```python
from build123d import *

# Parameters (mm, degrees)
F1_DEPTH = 6.35
F2_R     = 3.175
F3_DEPTH = 6.35
F5_DEPTH = 6.35
F4_R     = 22.225
F4_R_2   = 19.05
F6_DEPTH = 25.4


with BuildPart() as f1:
    # F0 (on Top) → F1 (new body)
    with BuildSketch(Plane.XY):
        Polygon((-42.868439, 12.7), (-42.868439, 0), (-42.868439, -12.7), (58.731561, -12.7), (58.731561, 12.7), align=None)
    extrude(amount=F1_DEPTH)

    # F2 (on face) → F3 (cut)
    with BuildSketch(Plane.XY.offset(6.35)):
        with Locations((33.331561, 0)):
            Circle(F2_R)
    extrude(amount=-F3_DEPTH, mode=Mode.SUBTRACT)

    # F4 (on face) → F5 (join)
    with BuildSketch(Plane.XY.offset(6.35)):
        with BuildLine():
            ThreePointArc((77.781561, 0), (65.529022, 17.795983), (44.532529, 12.7))
            Line((44.532529, 12.7), (58.731561, 12.7))
            Line((58.731561, 12.7), (58.731561, -12.7))
            Line((58.731561, -12.7), (44.532529, -12.7))
            ThreePointArc((44.532529, -12.7), (65.529022, -17.795983), (77.781561, 0))
        make_face()
        with BuildLine():
            Line((58.731561, 12.7), (44.532529, 12.7))
            ThreePointArc((44.532529, 12.7), (39.681561, 0), (44.532529, -12.7))
            Line((44.532529, -12.7), (58.731561, -12.7))
            Line((58.731561, -12.7), (58.731561, 12.7))
        make_face()
    extrude(amount=F5_DEPTH)

    # F4 (on face) → F6 (join)
    with BuildSketch(Plane.XY.offset(6.35)):
        with Locations((58.731561, 0)):
            Circle(F4_R)
        with Locations((58.731561, 0)):
            Circle(F4_R_2, mode=Mode.SUBTRACT)
    extrude(amount=F6_DEPTH)


solid = f1.part
```
Geometry: final body of the model. Coordinates: model frame, mm. A direction names the side the tool comes from. Coordinates: 2 decimals unless noted, no trailing zeros. Loops run counter-clockwise (first coordinate to the right, second up) from the corner with the lowest first, then second, coordinate; pieces in that order, holes last. Notation, with made-up numbers: (18.5, 34) -> (70.5, 34) arc R21 cw to (70.5, 71) -> close; hole circle Ø8 at (11.5, 56.25). An arc over 180 degrees is marked (long way). Use a Markdown table: item, result. Add a question column.
(1) Section query C-C, the plane y = 5. Return loops of the section in (x, z).
(2) Pin query (flat end, axial travel): pin 1 Ø23 at (x, y) = (58.73, 0) entering from +Z; pin 2 Ø12 at (x, y) = (-18, -9.5) entering from +Z; pin 3 Ø6 at (x, z) = (1.5, 7.5) entering from +Y; pin 4 Ø1 at (x, y) = (29, -5.5) entering from -Z. Return the tip coordinate at first contact, or that it passes through.
(3) Access query for faces 5 (the flat face through (58, 0, 12.7)), 6 (the flat face through (7, 0, 0)), 7 (the flat face through (9, 12.7, 3)), 8 (the flat face through (-42.868, 0, 3)), 9 (the flat face through (58.732, 0, 3)). Directions: +Z, -Z, +X, -X, +Y, -Y. A direction counts if a zero-diameter tool reaches every point of the face in a straight line with its end or side. Return the directions, or none.
(4) Mould query, pull axis Y, two halves, no side actions, for faces 1 (the cylindrical face through (36.53, 0.98, 18.87)), 2 (the flat face through (65, 0, 6.35)), 3 (the cylindrical face through (30.16, 0.14, 3.22)), 4 (the flat face through (7, -12.7, 3)). Classes: pulls with the +Y half, pulls with the -Y half, needs draft (parallel to the pull), parting line crosses it, or undercut.
(5) Section query B-B, the plane x = 72.5. Return loops of the section in (y, z), plus the area to 3 significant figures.
(6) Section query A-A, the plane z = 27. Return loops of the section in (x, y) (3 decimals).
(7) Section query D-D, the plane x = 49. Return loops of the section in (y, z), plus the area to 3 significant figures.
(8) Line query: line 1 along X through (y, z) = (0, 21.5); line 2 along Z through (x, y) = (3, 7); line 3 along Z through (x, y) = (69.5, 17). Output: solid intervals per line, ascending.
Answer:
| question | item | result |
|---|---|---|
| 1 | outline | (-42.87, 0) -> (58.73, 0) -> (58.73, 6.35) -> (80.39, 6.35) -> (80.39, 31.75) -> (77.11, 31.75) -> (77.11, 12.7) -> (40.35, 12.7) -> (40.35, 31.75) -> (37.08, 31.75) -> (37.08, 6.35) -> (-42.87, 6.35) -> close |
| 2 | pin 1 | stops at z = 12.7 |
| 2 | pin 2 | stops at z = 6.35 |
| 2 | pin 3 | stops at y = 12.7 |
| 2 | pin 4 | stops at z = 0 |
| 3 | face 5 | +Z |
| 3 | face 6 | -Z, +X, -X, +Y, -Y |
| 3 | face 7 | -Z, +X, -X, +Y |
| 3 | face 8 | +Z, -Z, -X, +Y, -Y |
| 3 | face 9 | -Z, +X, +Y, -Y |
| 4 | face 1 | parting line crosses it |
| 4 | face 2 | needs draft |
| 4 | face 3 | undercut |
| 4 | face 4 | pulls with the -Y half |
| 5 | outline | (-17.45, 6.35) -> (17.45, 6.35) -> (17.45, 31.75) -> (13.17, 31.75) -> (13.17, 12.7) -> (-13.17, 12.7) -> (-13.17, 31.75) -> (-17.45, 31.75) -> close |
| 5 | area | 385 mm^2 |
| 6 | outline | circle Ø44.45 at (58.732, 0); hole circle Ø38.1 at (58.732, 0) |
| 7 | outline | (-19.98, 6.35) -> (-12.7, 6.35) -> (-12.7, 0) -> (12.7, 0) -> (12.7, 6.35) -> (19.98, 6.35) -> (19.98, 31.75) -> (16.38, 31.75) -> (16.38, 12.7) -> (-16.38, 12.7) -> (-16.38, 31.75) -> (-19.98, 31.75) -> close |
| 7 | area | 552 mm^2 |
| 8 | line 1 | x = 36.51 to 39.68, 77.78 to 80.96 |
| 8 | line 2 | z = 0 to 6.35 |
| 8 | line 3 | z = 6.35 to 31.75 |
